The model under review builds one solid part; all positions refer to its coordinate system, in mm. Face numbers are marked on the shaded views. A direction names the side the tool comes from. Give positions to 0.01 mm unless a question says otherwise; leave off trailing zeros. Order: outer loops, then holes, each group sorted by start corner. A loop starts at its lowest first (then second) coordinate and runs counter-clockwise, first axis right, second up. Notation, with made-up numbers: (-16, 65.5) - (-5, 65.5) arc R24 ccw to (-5, 76.5) - close; hole circle Ø4 at (41, 26). An arc over 180 degrees is marked (long way). Use CSV: the item, a comma, the result in double quotes.
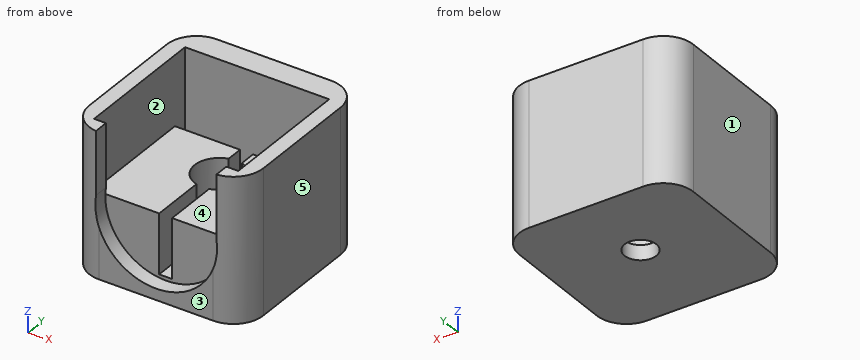
```python
from build123d import *

# Parameters (mm, degrees)
F1_DEPTH  = 1.5
F2_W      = 13.5
F2_H      = 14.5
F2_W_2    = 1.5
F3_DEPTH  = 1.5
F4_W      = 1.5
F4_H      = 14.5
F4_W_2    = 13.5
F5_DEPTH  = 1.5
F6_W      = 16
F6_H      = 14.5
F6_W_2    = 1.5
F7_DEPTH  = 2.5
F8_W      = 14.5
F8_H      = 13.5
F9_DEPTH  = 1.5
F10_W     = 12
F10_H     = 6
F11_DEPTH = 14.5
F12_W     = 1.3
F12_H     = 12
F13_DEPTH = 6
F14_R     = 2.5
F14_R_2   = 1.6
F15_DEPTH = 13
F16_DEPTH = 14.5010001
F17_R     = 3


with BuildPart() as f1:
    # F0 (on Front) → F1 (new body)
    with BuildSketch(Plane.XZ):
        with BuildLine():
            Line((-6.0567391277, 7.25), (-7.25, 7.25))
            Line((-7.25, 7.25), (-7.25, -7.25))
            Line((-7.25, -7.25), (7.25, -7.25))
            Line((7.25, -7.25), (7.25, 7.25))
            Line((7.25, 7.25), (6.0567391277, 7.25))
            Line((6.0567391277, 7.25), (6.0567391277, 0.9118860342))
            add(Edge.make_bspline(
                [(6.125, 0), (6.125, 0.4584979124), (6.0567391277, 0.9118860342)],
                knots=[0, 0, 0, 0.1494348984, 0.1494348984, 0.1494348984], degree=2, weights=[1, 0.9972099498, 1]))
            add(Edge.make_bspline(
                [(-6.0567391277, 0.9118860342), (-7.0394373604, -5.6151871016), (-0.4572186802, -6.1079109423), (6.125, -6.6006347829), (6.125, 0)],
                knots=[2.9921577552, 2.9921577552, 2.9921577552, 4.6376715312, 4.6376715312, 6.2831853072, 6.2831853072, 6.2831853072], degree=2, weights=[1, 0.6802029301, 1, 0.6802029301, 1]))
            Line((-6.0567391277, 0.9118860342), (-6.0567391277, 7.25))
        make_face()
    extrude(amount=F1_DEPTH)

    # F2 (on face) → F3 (join)
    with BuildSketch(Plane.YZ.offset(7.25)):
        with Locations((6.75, 0)):
            Rectangle(F2_W, F2_H)
        with Locations((-0.75, 0)):
            Rectangle(F2_W_2, F2_H)
    extrude(amount=F3_DEPTH)

    # F4 (on face) → F5 (join)
    with BuildSketch(Plane(origin=(-7.25, 0, 0), x_dir=(0, -1, 0), z_dir=(-1, 0, 0))):
        with Locations((0.75, 0)):
            Rectangle(F4_W, F4_H)
        with Locations((-6.75, 0)):
            Rectangle(F4_W_2, F4_H)
    extrude(amount=F5_DEPTH)

    # F6 (on face) → F7 (join)
    with BuildSketch(Plane(origin=(0, 13.5, 0), x_dir=(-1, 0, 0), z_dir=(0, 1, 0))):
        with Locations((-0.75, 0)):
            Rectangle(F6_W, F6_H)
        with Locations((8, 0)):
            Rectangle(F6_W_2, F6_H)
    extrude(amount=F7_DEPTH)

    # F8 (on face) → F9 (join)
    with BuildSketch(Plane(origin=(0, 0, -7.25), x_dir=(1, 0, 0), z_dir=(0, 0, -1))):
        with Locations((0, -6.75)):
            Rectangle(F8_W, F8_H)
    extrude(amount=-F9_DEPTH)

    # F10 (on face) → F11 (join, through all)
    with BuildSketch(Plane.YZ.offset(-7.25)):
        with Locations((6, -2.75)):
            Rectangle(F10_W, F10_H)
    extrude(amount=F11_DEPTH)

    # F12 (on face) → F13 (cut, through all)
    with BuildSketch(Plane.XY.offset(0.25)):
        with Locations((-0.051082634, 6)):
            Rectangle(F12_W, F12_H)
    extrude(amount=-F13_DEPTH, mode=Mode.SUBTRACT)

    # F14 (on face) → F15 (cut, through all)
    with BuildSketch(Plane.XY.offset(7.25)):
        with Locations((0, 7.9200456385)):
            Circle(F14_R)
        with Locations((0, 7.9200456385)):
            Circle(F14_R_2, mode=Mode.SUBTRACT)
    extrude(amount=-F15_DEPTH, mode=Mode.SUBTRACT)

    # F14 (on face) → F16 (cut, through all)
    with BuildSketch(Plane.XY.offset(7.25)):
        with Locations((0, 7.9200456385)):
            Circle(F14_R_2)
    extrude(amount=-F16_DEPTH, mode=Mode.SUBTRACT)

    # F17
    f17_edges = [f1.edges().sort_by_distance(p)[0] for p in [
        (8.75, -1.5, 0),
        (-8.75, -1.5, 0),
        (-8.75, 16, 0),
        (8.75, 16, 0),
    ]]
    fillet(f17_edges, radius=F17_R)


solid = f1.part
```
Item 1: Mouldability with a two-part tool opening along Y and no side actions: class the marked faces 1, 2 and 3 as pulls with the +Y half, pulls with the -Y half, needs draft (parallel to the pull), parting line crosses it, or undercut.
Results list:
face 1,"needs draft"
face 2,"undercut"
face 3,"pulls with the -Y half"
Item 2: Take a section at C-C, the plane z = 1.25. Give the boundary of the cut face in (x, y).
Results list:
outline,"(-8.75, 1.5) arc R3 ccw to (-6.06, -1.48) - (-6.06, 0) - (-7.25, 0) - (-7.25, 13.5) - (7.25, 13.5) - (7.25, 0) - (6.06, 0) - (6.06, -1.48) arc R3 ccw to (8.75, 1.5) - (8.75, 13) arc R3 ccw to (5.75, 16) - (-5.75, 16) arc R3 ccw to (-8.75, 13) - close"
Item 3: Wall thickness on L1, parallel to X at y = 3.25, z = 4.75; L2, parallel to X at y = 11.25, z = 0; L3, parallel to Y at x = 5.75, z = -3.25: over which ranges is each line inside the solid? List them lowest first.
Results list:
L1,"x = -8.75 to -7.25, 7.25 to 8.75"
L2,"x = -8.75 to -0.7, 0.6 to 8.75"
L3,"y = -1.5 to 12, 13.5 to 16"
Item 4: Take a section at D-D, the plane y = 0.5. Give the boundary of the cut face in (x, z), and give its area (3 significant figures).
Results list:
outline,"(-8.58, -7.25) - (8.58, -7.25) - (8.58, 7.25) - (7.25, 7.25) - (7.25, 0.25) - (0.6, 0.25) - (0.6, -5.75) - (-0.7, -5.75) - (-0.7, 0.25) - (-7.25, 0.25) - (-7.25, 7.25) - (-8.58, 7.25) - close"
area,"139 mm2"
Item 5: Take a section at B-B, the plane y = 11.5. Give the boundary of the cut face in (x, z), and give its area (3 significant figures).
Results list:
outline,"(-8.75, -7.25) - (8.75, -7.25) - (8.75, 7.25) - (7.25, 7.25) - (7.25, 0.25) - (0.6, 0.25) - (0.6, -5.75) - (-0.7, -5.75) - (-0.7, 0.25) - (-7.25, 0.25) - (-7.25, 7.25) - (-8.75, 7.25) - close"
area,"144 mm2"
Item 6: Tool access review of the marked faces 4 and 5: name each direction out of +Z, -Z, +X, -X, +Y, -Y from which nothing blocks a thin tool from reaching the whole face with its end or side.
Results list:
face 4,"+Z"
face 5,"+Z, -Z, +X, +Y, -Y"
Item 7: Clearance check with flat-ended pins moving along their axes: pin 1 (1 mm diameter, centred on x = 2, y = 9, fed in from +Z); pin 2 (1.3 mm diameter, centred on x = 7, z = 4, fed in from +Y); pin 3 (6.5 mm diameter, centred on x = 1, z = 2, fed in from -Y). State where each tip first meets the part, or that it passes through.
Results list:
pin 1,"stops at z = 0.25"
pin 2,"stops at y = 15.94"
pin 3,"stops at y = 0"
Item 8: Take a section at A-A, the plane y = 9. Give the boundary of the cut face in (x, z), and give its area (3 significant figures).
Results list:
outline,"(-8.75, -7.25) - (-1.18, -7.25) - (-1.18, -5.75) - (-2.25, -5.75) - (-2.25, 0.25) - (-7.25, 0.25) - (-7.25, 7.25) - (-8.75, 7.25) - close; (1.18, -7.25) - (8.75, -7.25) - (8.75, 7.25) - (7.25, 7.25) - (7.25, 0.25) - (2.25, 0.25) - (2.25, -5.75) - (1.18, -5.75) - close"
area,"122 mm2"
